```python
from build123d import *

# Parameters (mm, degrees)
SKETCH1_W           = 120
SKETCH1_H           = 60
BOSS_EXTRUDE1_DEPTH = 20
CUT_EXTRUDE1_DEPTH  = 20
BOSS_EXTRUDE2_DEPTH = 10


with BuildPart() as part:
    # Sketch1 → Boss-Extrude1 (new body)
    with BuildSketch(Plane(origin=(0, 0, 0), x_dir=(0, 0, -1), z_dir=(1, 0, 0))):
        Rectangle(SKETCH1_W, SKETCH1_H)
    extrude(amount=BOSS_EXTRUDE1_DEPTH)

    # Sketch3 → Cut-Extrude1 (cut)
    with BuildSketch(Plane.ZY):
        Polygon((45, 0), (60, -15), (60, 15), align=None)
    cut_extrude1 = extrude(amount=-CUT_EXTRUDE1_DEPTH, mode=Mode.SUBTRACT)

    # Mirror4: Cut-Extrude1 across plane
    add(cut_extrude1.mirror(Plane(origin=(0, 0, 0), x_dir=(1, 0, 0), z_dir=(0, 0, -1))), mode=Mode.SUBTRACT)

    # Sketch4 → Boss-Extrude2 (add, symmetric)
    with BuildSketch(Plane.XY):
        Polygon((20, 30), (60, 30), (60, 15), (45, 0), (60, -15), (60, -30), (20, -30), align=None)
    extrude(amount=BOSS_EXTRUDE2_DEPTH, both=True)


solid = part.part
```
Verification items for the finished model (mm, model axes). A direction names the side the tool comes from. Coordinates: 2 decimals unless noted, no trailing zeros. Loops run counter-clockwise (first coordinate to the right, second up) from the corner with the lowest first, then second, coordinate; pieces in that order, holes last. Notation, with made-up numbers: (44.5, 65) -> (99.5, 65) arc R20 cw to (99.5, 87) -> close; hole circle Ø1 at (64.5, -35). An arc over 180 degrees is marked (long way). Put each result on its own line as item: value.
1. Section check B-B, the plane x = 56. Record the boundary of the cut face in (y, z), then the cut area to 3 significant figures.
Result set:
outline: (-30, -10) -> (-11, -10) -> (-11, 10) -> (-30, 10) -> close; (11, -10) -> (30, -10) -> (30, 10) -> (11, 10) -> close
area: 760 mm^2
2. Section check A-A, the plane z = 51.5. Record the boundary of the cut face in (x, y), then the cut area to 3 significant figures.
Result set:
outline: (0, -30) -> (20, -30) -> (20, -6.5) -> (0, -6.5) -> close; (0, 6.5) -> (20, 6.5) -> (20, 30) -> (0, 30) -> close
area: 940 mm^2
3. Gauge pin test, flat ends, axial feed: P1, Ø3, axis at x = 37.5, y = 22.5, coming from the -Z side; P2, Ø3, axis at y = -0.5, z = -8, coming from the +X side; P3, Ø25, axis at y = 2.5, z = -40.5, coming from the +X side. Record the tip position at first contact, or that the pin passes through.
Result set:
P1: stops at z = -10
P2: stops at x = 47
P3: stops at x = 20
4. Tool access check on faces 5 (the face through (40, 0, 10)), 6 (the face through (10, -7, 52)), 7 (the face through (52, -7, 0)), 8 (the face through (40, 0, -10)), 9 (the face through (10, -7, -52)). Record the directions out of +Z, -Z, +X, -X, +Y, -Y that give a thin tool (end or side, any length) a straight path to the whole face; none if there is none.
Result set:
face 5: +Z, +X, +Y, -Y
face 6: +Z, +X, -X
face 7: +Z, -Z, +X
face 8: -Z, +X, +Y, -Y
face 9: -Z, +X, -X
5. Mould release check, pull along Y, two halves, no side actions. Record for faces 1 (the face through (16, -30, 1)), 2 (the face through (10, 8, -53)), 3 (the face through (20, 0, -35)), 4 (the face through (16, 30, 1)): pulls with the +Y half, pulls with the -Y half, needs draft (parallel to the pull), parting line crosses it, or undercut.
Result set:
face 1: pulls with the -Y half
face 2: undercut
face 3: needs draft
face 4: pulls with the +Y half
6. Section check D-D, the plane x = 11. Record the boundary of the cut face in (y, z).
Result set:
outline: (-30, -60) -> (-15, -60) -> (0, -45) -> (15, -60) -> (30, -60) -> (30, 60) -> (15, 60) -> (0, 45) -> (-15, 60) -> (-30, 60) -> close
7. Thickness scan on line 1 (Z direction, x = 35, y = -18); line 2 (X direction, y = 21.5, z = -19); line 3 (Z direction, x = 18, y = 10). Record the ranges inside material, lowest first.
Result set:
line 1: z = -10 to 10
line 2: x = 0 to 20
line 3: z = -55 to 55
8. Section check C-C, the plane y = -7.5. Record the boundary of the cut face in (x, z).
Result set:
outline: (0, -52.5) -> (20, -52.5) -> (20, -10) -> (52.5, -10) -> (52.5, 10) -> (20, 10) -> (20, 52.5) -> (0, 52.5) -> close
